Here's the drawing with two shaded views (mm, measured from the low corner). I have some questions. Round coordinates to 2 decimals unless told otherwise and drop trailing zeros. Loops run counter-clockwise (first coordinate to the right, second up) from the corner with the lowest first, then second, coordinate; pieces in that order, holes last. Notation, with made-up numbers: M 80.25,17 L 126.25,17 A18 cw 126.25,37 Z; hole C 14.5,-30.5 d8. An arc over 180 degrees is marked long. Answer as a JSON object with one key per item and string values.
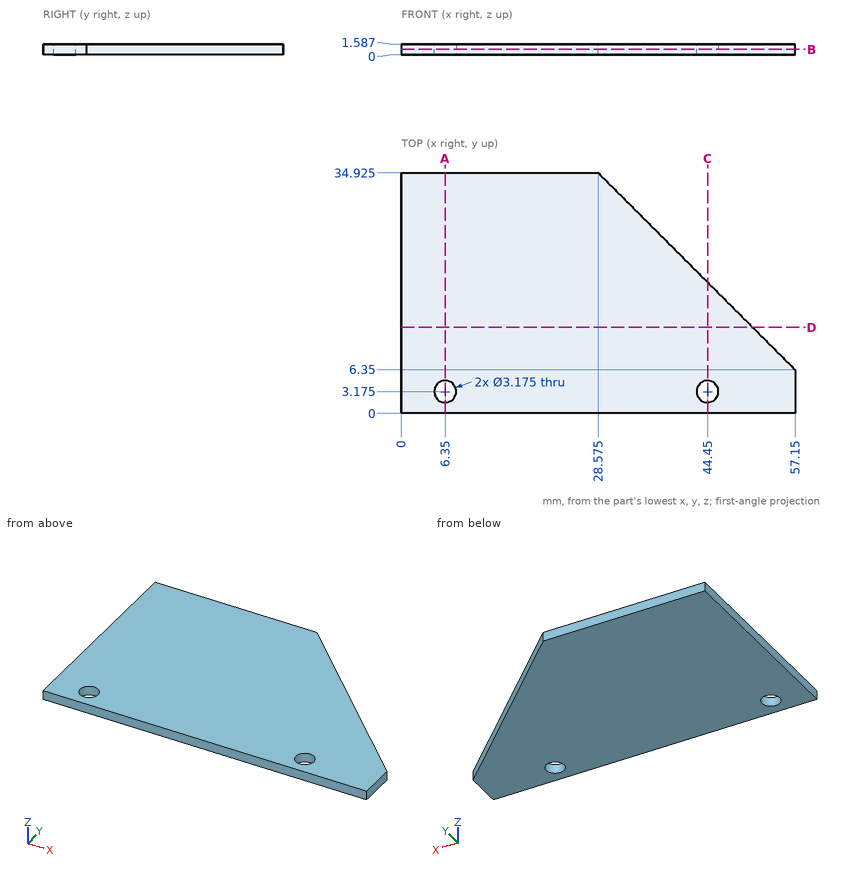
Item 1: For P1, Ø3.5, axis at x = 44.45, y = 3.175, coming from the +Z side; P2, Ø3, axis at x = 6.35, y = 3.175, coming from the -Z side, each with a flat end and sliding along its axis, tell me the tip position at first contact or that it passes through.
Solution:
{"P1": "stops at z = 1.59", "P2": "passes through"}
Item 2: I want a section at C-C on x = 44.45. List the corners of the cut face in (y, z) for me, plus the area to 3 significant figures.
Solution:
{"outline": "M 0,0 L 1.59,0 L 1.59,1.59 L 0,1.59 Z; M 4.76,0 L 19.05,0 L 19.05,1.59 L 4.76,1.59 Z", "area": "25.2 mm2"}
Item 3: I want a section at B-B on z = 0.8. Count the separate pieces of the cut face and the enclosed holes in it, plus the area to 3 significant figures.
Solution:
{"separate pieces": "1", "enclosed holes": "2", "area": "1,570 mm2"}
Item 4: If I drill on L1, parallel to Y at x = 6.35, z = 0.95 (1 decimal); L2, parallel to Y at x = 45, z = 0.3 (1 decimal); L3, parallel to X at y = 21, z = 0.25, over which ranges is the centre line in solid material (lowest first)? Write a range as from..to.
Solution:
{"L1": "y = 0..1.6, 4.8..34.9", "L2": "y = 0..1.7, 4.7..18.5", "L3": "x = 0..42.5"}
Item 5: I want a section at A-A on x = 6.35. List the corners of the cut face in (y, z) for me (1 decimal).
Solution:
{"outline": "M 0,0 L 1.6,0 L 1.6,1.6 L 0,1.6 Z; M 4.8,0 L 34.9,0 L 34.9,1.6 L 4.8,1.6 Z"}
Item 6: I want a section at D-D on y = 12.5. List the corners of the cut face in (x, z) for me.
Solution:
{"outline": "M 0,0 L 51,0 L 51,1.59 L 0,1.59 Z"}
